The listing builds one solid part. Answer for the finished solid, in the listing's coordinates (mm). A direction names the side the tool comes from. Round coordinates to 2 decimals unless told otherwise and drop trailing zeros. Write each loop counter-clockwise with the first axis right and the second up, starting at its lowest first coordinate (ties: lowest second). Pieces come first, ordered by that corner, then holes.
from build123d import *

# Parameters (mm, degrees)
F0_R     = 10
F1_DEPTH = 30
F2_R     = 10
F2_R_2   = 9
F2_R_3   = 8
F3_DEPTH = 2


with BuildPart() as f1:
    # F0 (on Top) → F1 (new body)
    with BuildSketch(Plane.XY):
        Circle(F0_R)
    extrude(amount=F1_DEPTH)

    # F2 (on face) → F3 (join)
    with BuildSketch(Plane.XY.offset(30)):
        Circle(F2_R)
        Circle(F2_R_2, mode=Mode.SUBTRACT)
        Circle(F2_R_3)
        with BuildLine():
            Line((-3.5, 4.0707142143), (3.5, 4.0707142143))
            ThreePointArc((3.5, 4.0707142143), (3.9609772229, 3.7643633816), (3.8570714214, 3.2207142143))
            Line((3.8570714214, 3.2207142143), (0.5, -0.2041836837))
            Line((0.5, -0.2041836837), (0.5, -3.5))
            Line((0.5, -3.5), (1.5, -3.5))
            ThreePointArc((1.5, -3.5), (2, -4), (1.5, -4.5))
            Line((1.5, -4.5), (0, -4.5))
            Line((0, -4.5), (-1.5, -4.5))
            ThreePointArc((-1.5, -4.5), (-2, -4), (-1.5, -3.5))
            Line((-1.5, -3.5), (-0.5, -3.5))
            Line((-0.5, -3.5), (-0.5, -0.2041836837))
            Line((-0.5, -0.2041836837), (-3.8570714214, 3.2207142143))
            ThreePointArc((-3.8570714214, 3.2207142143), (-3.9609772229, 3.7643633816), (-3.5, 4.0707142143))
        make_face(mode=Mode.SUBTRACT)
        Polygon((0, 0.7142857143), (2.3097619286, 3.0707142143), (-2.3097619286, 3.0707142143), align=None)
    extrude(amount=F3_DEPTH)


solid = f1.part
1. For a pull along Y with two mould halves and no side action, classify faces 3 (the face through (-0.5, -2, 31)), 4 (the face through (-9, 2, 32)) as released by +Y, released by -Y, zero draft, split by the parting line, or undercut.
Geometry says:
face 3: undercut
face 4: zero draft
2. Section D-D on y = -4 is taken. Determine the outline of the cut face in (x, z).
Geometry says:
outline: (-9.17, 0) - (9.17, 0) - (9.17, 32) - (8.06, 32) - (8.06, 30) - (6.93, 30) - (6.93, 32) - (2, 32) - (2, 30) - (-2, 30) - (-2, 32) - (-6.93, 32) - (-6.93, 30) - (-8.06, 30) - (-8.06, 32) - (-9.17, 32) - close
3. Section A-A on y = 6 is taken. Determine the outline of the cut face in (x, z).
Geometry says:
outline: (-8, 0) - (8, 0) - (8, 32) - (6.71, 32) - (6.71, 30) - (5.29, 30) - (5.29, 32) - (-5.29, 32) - (-5.29, 30) - (-6.71, 30) - (-6.71, 32) - (-8, 32) - close
4. Straight lines are drawn through the part: line 1 along Y through (x, z) = (-3, 31); line 2 along Z through (x, y) = (8.5, 2.75); line 3 along X through (y, z) = (3, 10). For each, find the intervals that lie inside material, in ascending order.
Geometry says:
line 1: y = -9.54 to -8.49, -7.42 to 2.35, 4.07 to 7.42, 8.49 to 9.54
line 2: z = 0 to 30
line 3: x = -9.54 to 9.54
5. Section B-B on x = -5.75 is taken. Determine the outline of the cut face in (y, z).
Geometry says:
outline: (-8.18, 0) - (8.18, 0) - (8.18, 32) - (6.92, 32) - (6.92, 30) - (5.56, 30) - (5.56, 32) - (-5.56, 32) - (-5.56, 30) - (-6.92, 30) - (-6.92, 32) - (-8.18, 32) - close
6. A tool of negligible diameter and unlimited length cuts with its end or side. For faces 1 (the face through (2, 0, 32)), 2 (the face through (2.2, 1.53, 30.99)), from which of +Z, -Z, +X, -X, +Y, -Y can it reach the whole face along a straight path? Write none if from no direction.
Geometry says:
face 1: +Z, +X, -X, +Y, -Y
face 2: +Z
7. Given pin 1 (0.6 mm diameter, centred on x = -1, z = 31, fed in from +Y); pin 2 (2 mm diameter, centred on y = -1.5, z = 31, fed in from -X); pin 3 (1.5 mm diameter, centred on y = -7, z = 7, fed in from -X), each flat-ended and moving along its own axis, determine where each tip first touches the part or whether it passes through.
Geometry says:
pin 1: stops at y = 9.98
pin 2: stops at x = -9.99
pin 3: stops at x = -7.81
8. Section C-C on z = 10 is taken. Determine the outline of the cut face in (x, y), plus the area to 3 significant figures.
Geometry says:
outline: circle Ø20 at (0, 0)
area: 314 mm2
